Autodesk Fusion 360 part; units mm, degrees
sketch "Sketch1" plane through (0, 0, 0) normal (0, 0, 1) x (1, 0, 0)
  line L0 (0, -50) -> (-40, -50)
  line L1 (-40, -50) -> (-40, 0)
  line L2 (-40, 0) -> (0, 0)
  line L3 (0, 0) -> (0, -50)
extrude "Extrude1" add sketch "Sketch1" along normal blind 8
sketch "Sketch2" plane through (0, 0, 8) normal (0, 0, 1) x (-1, 0, 0)
  line L0 (0, 0) -> (40, 0)
  line L1 (40, 0) -> (40, 50)
  line L2 (40, 50) -> (0, 50)
  line L3 (0, 50) -> (0, 0)
  line L4 (21, 0) -> (16, 0)
  line L5 (16, 0) -> (16, 20)
  line L6 (16, 20) -> (21, 20)
  line L7 (21, 20) -> (21, 0)
  dimension "d3" = 5
  dimension "d4" = 20
extrude "Extrude2" add sketch "Sketch2" along normal blind 25 contours L0 L4 L5 L6 L7
hole "Hole1" at (-16, -12.5, 11) direction (-1, 0, 0) diameter 3 depth 6 tip angle 118
hole "Hole2" at (-16, -12.5, 28) direction (-1, 0, 0) diameter 3 depth 6 tip angle 118
hole "Hole3" at (-16, -6, 20) direction (-1, 0, 0) diameter 4.2 depth 6 tip angle 118
extrude "Extrude3" cut 1 faces at (-13.3333, -33.3333, 0) along direction (0, 0, 1) blind 8
The model under review builds one solid part; all positions refer to its coordinate system, in mm. Give positions to 0.01 mm unless a question says otherwise; leave off trailing zeros. Write each loop counter-clockwise with the first axis right and the second up, starting at its lowest first coordinate (ties: lowest second). Pieces come first, ordered by that corner, then holes.
1. Draft analysis for pull direction Y (two halves, no side actions). For faces 1 (the flat face through (-18, -20, 20)), 2 (the cylindrical face through (-18.535, -6.631, 17.997)), 3 (the flat face through (-21, -10, 20)), state which applies: +Y half, -Y half, draft (parallel to the pull), parting line (faces both ways), or undercut.
2. Wall thickness on L1, parallel to Z at x = -19.35, y = -12.5; L2, parallel to Y at x = -19.3, z = 28; L3, parallel to Z at x = -17.4, y = -12: over which ranges is each line inside the solid? List them lowest first.
3. Add section D-D, the plane y = -6. Write out the cut boundary in (x, z).
4. Add section B-B, the plane y = -12.5. Write out the cut boundary in (x, z).
5. For P1, Ø3.5, axis at y = -6, z = 20, coming from the +X side, flat-tipped, find the tip position at first contact; note if it passes through.
6. Add section C-C, the plane x = -19.7. Write out the cut boundary in (y, z).
7. Add section A-A, the plane z = 11. Write out the cut boundary in (x, y), plus the area to 3 significant figures.
Worked answers:
1. face 1: -Y half
1. face 2: undercut
1. face 3: draft
2. L1: z = 8 to 9.5, 12.5 to 26.5, 29.5 to 33
2. L2: y = -20 to -14, -11 to 0
2. L3: z = 8 to 9.59, 12.41 to 26.59, 29.41 to 33
3. outline: (-21, 8) - (-16, 8) - (-16, 17.9) - (-21, 17.9) - close; (-21, 22.1) - (-16, 22.1) - (-16, 33) - (-21, 33) - close
4. outline: (-21, 8) - (-16, 8) - (-16, 9.5) - (-21, 9.5) - close; (-21, 12.5) - (-16, 12.5) - (-16, 26.5) - (-21, 26.5) - close; (-21, 29.5) - (-16, 29.5) - (-16, 33) - (-21, 33) - close
5. P1: passes through
6. outline: (-20, 8) - (0, 8) - (0, 33) - (-20, 33) - close; hole circle Ø3 at (-12.5, 11); hole circle Ø3 at (-12.5, 28); hole circle Ø4.2 at (-6, 20)
7. outline: (-21, -20) - (-16, -20) - (-16, -14) - (-21, -14) - close; (-21, -11) - (-16, -11) - (-16, 0) - (-21, 0) - close
7. area: 85.0 mm2
